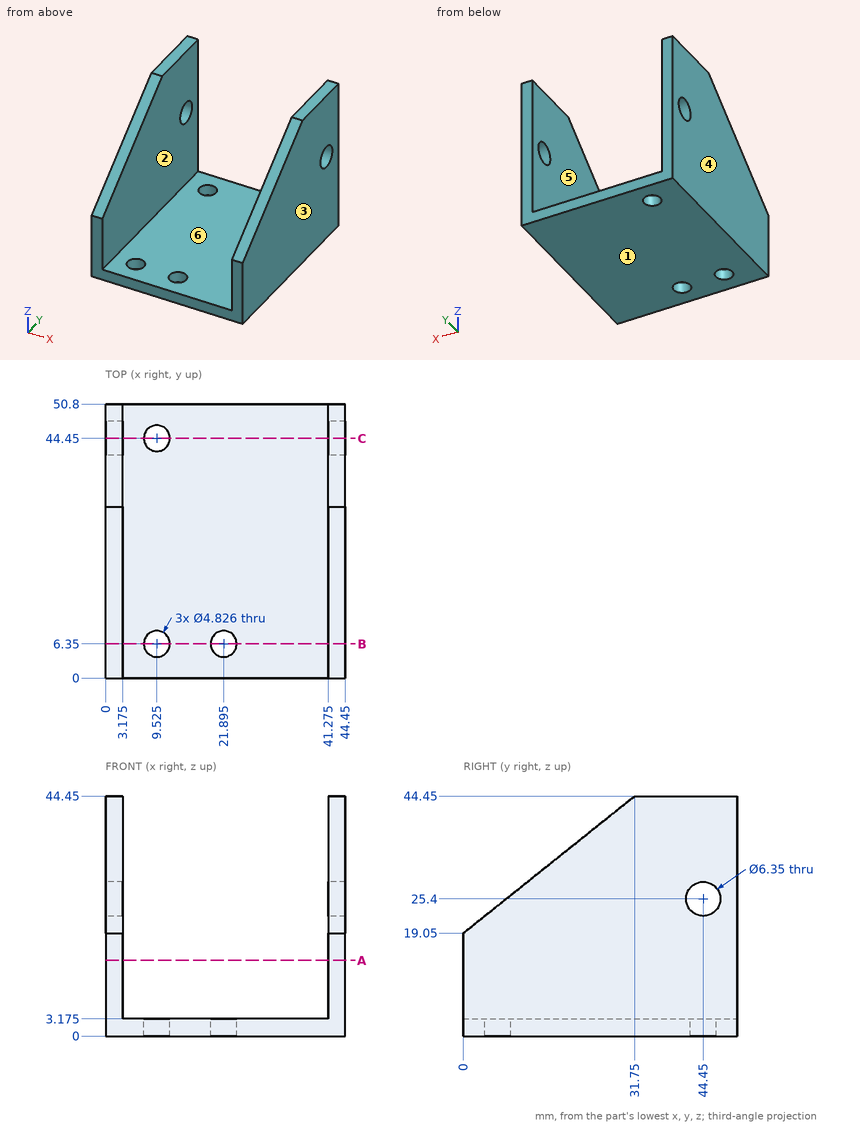
Part print with two shaded views. Sizes in mm from the minimum x, y, z corner. A direction names the side the tool comes from. Give positions to 0.01 mm unless a question says otherwise; leave off trailing zeros. Order: outer loops, then holes, each group sorted by start corner. A loop starts at its lowest first (then second) coordinate and runs counter-clockwise, first axis right, second up.
1) 3-axis set-ups, long thin cutter, end or side, ignore diameter. For the marked faces 1 and 2: which of +Z, -Z, +X, -X, +Y, -Y reach the whole face in a straight line?
2) Mould opens along X. For the marked faces 3, 4, 5 and 6 say: +X half, -X half, draft (parallel to the pull), parting line (faces both ways), or undercut.
3) Saw through at A-A, the plane z = 14. Write the cut outline in (x, y) (3 decimals).
4) Saw through at C-C, the plane y = 44.45. Write the cut outline in (x, z) (3 decimals).
5) Wall check: probe 1 along X at (y, z) = (6.35, 2.3); probe 2 along X at (y, z) = (44.45, 2.05); probe 3 along X at (y, z) = (34.5, 31) (3 decimals). Give the ranges that are in metal, low to high.
6) Saw through at B-B, the plane y = 6.35. Count the separate pieces of the cut face and the enclosed holes in it.
7) Pin check, flat tips, straight feed: pin 1 (3 mm diameter, centred on x = 6.5, z = 9.5, fed in from -Y); pin 2 (4 mm diameter, centred on x = 37, y = 33, fed in from +Z) (3 decimals). Stop position of each tip, or through.
Computed:
1. face 1: -Z, +X, -X, +Y, -Y
1. face 2: +Z, +Y, -Y
2. face 3: +X half
2. face 4: -X half
2. face 5: undercut
2. face 6: undercut
3. outline: (0, 0) - (3.175, 0) - (3.175, 50.8) - (0, 50.8) - close; (41.275, 0) - (44.45, 0) - (44.45, 50.8) - (41.275, 50.8) - close
4. outline: (0, 0) - (7.112, 0) - (7.112, 3.175) - (3.175, 3.175) - (3.175, 22.225) - (0, 22.225) - close; (0, 28.575) - (3.175, 28.575) - (3.175, 44.45) - (0, 44.45) - close; (11.938, 0) - (44.45, 0) - (44.45, 22.225) - (41.275, 22.225) - (41.275, 3.175) - (11.938, 3.175) - close; (41.275, 28.575) - (44.45, 28.575) - (44.45, 44.45) - (41.275, 44.45) - close
5. probe 1: x = 0 to 7.11, 11.94 to 19.48, 24.31 to 44.45
5. probe 2: x = 0 to 7.11, 11.94 to 44.45
5. probe 3: x = 0 to 3.175, 41.275 to 44.45
6. separate pieces: 3
6. enclosed holes: 0
7. pin 1: passes through
7. pin 2: stops at z = 3.175
